```python
from build123d import *

# Parameters (mm, degrees)
F0_W     = 50.8
F0_H     = 19.05
F1_DEPTH = 19.05
F2_R     = 5.08
F3_R     = 5.08
F4_W     = 18.7399210408
F4_H     = 7.62
F5_DEPTH = 0.508
F6_R     = 0.1690866305
F6_R_2   = 0.254
F6_R_3   = 0.1908338751
F6_R_4   = 0.1508847562
F7_DEPTH = 0.254
F8_W     = 6.35
F8_H     = 5.08
F9_DEPTH = 50.8
F10_R    = 5.07999


# Not quite as in the source:
# - a fillet or chamfer is up to 0.001 mm smaller than in the source, because OpenCascade refuses the exact size


with BuildPart() as f1:
    # F0 (on Top) → F1 (new body)
    with BuildSketch(Plane.XY):
        Rectangle(F0_W, F0_H)
    extrude(amount=F1_DEPTH)

    # F2
    f2_edges = [f1.edges().sort_by_distance(p)[0] for p in [
        (-25.4, -9.525, 9.525),
        (25.4, -9.525, 9.525),
    ]]
    fillet(f2_edges, radius=F2_R)

    # F3
    f3_edges = [f1.edges().sort_by_distance(p)[0] for p in [
        (25.4, 2.54, 0),
    ]]
    fillet(f3_edges, radius=F3_R)

    # F4 (on face) → F5 (join)
    with BuildSketch(Plane.XZ.offset(9.525)):
        with Locations((0.5450607277, 15.24)):
            Rectangle(F4_W, F4_H)
    extrude(amount=F5_DEPTH)

    # F6 (on face) → F7 (join)
    with BuildSketch(Plane.XZ.offset(10.033)):
        with Locations((4.971065205, 13.6094420754)):
            Circle(F6_R)
        with Locations((-3.7048892478, 13.6058607324)):
            Circle(F6_R_2)
        with Locations((5.0740026747, 16.8156122121)):
            Circle(F6_R_3)
        with Locations((-3.7048892478, 16.8490853095)):
            Circle(F6_R_4)
    extrude(amount=F7_DEPTH)

    # F8 (on face) → F9 (cut)
    with BuildSketch(Plane.YZ.offset(25.4)):
        with Locations((6.35, 16.51)):
            Rectangle(F8_W, F8_H)
    extrude(amount=-F9_DEPTH, mode=Mode.SUBTRACT)

    # F10 (radius 5.08 in the source; OpenCascade refuses exactly that, so slightly less here)
    f10_edges = [f1.edges().sort_by_distance(p)[0] for p in [
        (0, 3.175, 13.97),
    ]]
    fillet(f10_edges, radius=F10_R)


solid = f1.part
```
The listing builds one solid part. Answer for the finished solid, in the listing's coordinates (mm). A direction names the side the tool comes from. Give positions to 0.01 mm unless a question says otherwise; leave off trailing zeros. Order: outer loops, then holes, each group sorted by start corner. A loop starts at its lowest first (then second) coordinate and runs counter-clockwise, first axis right, second up.
1) Find section C-C on y = 5.5. Write down the section's boundary in (x, z).
Reported:
outline: (-25.4, 5.08) arc R5.08 ccw to (-20.32, 0) - (20.32, 0) arc R5.08 ccw to (25.4, 5.08) - (25.4, 14.78) - (-25.4, 14.78) - close
2) Find section B-B on z = 12.75. Write down the section's boundary in (x, y) (3 decimals), then the cut area to 3 significant figures.
Reported:
outline: (-25.4, -4.445) arc R5.08 ccw to (-20.32, -9.525) - (-8.825, -9.525) - (-8.825, -10.033) - (9.915, -10.033) - (9.915, -9.525) - (20.32, -9.525) arc R5.08 ccw to (25.4, -4.445) - (25.4, 9.525) - (-25.4, 9.525) - close
area: 966 mm2
3) For faces 1 (the face through (0, 9, 13.97)), 2 (the face through (23.872, 2.638, 1.449)), determine the directions among +Z, -Z, +X, -X, +Y, -Y from which every point of the face is accessible in a straight line to the end or side of a thin tool.
Reported:
face 1: +Z, +X, -X, +Y
face 2: -Z, +X, +Y, -Y
4) Consider line 1 along Y through (x, z) = (-19.5, 5.75) (3 decimals); line 2 along Z through (x, y) = (17, -5.25); line 3 along Y through (x, z) = (-9.5, 1) (3 decimals). Determine where each line is inside the solid, lowest interval first.
Reported:
line 1: y = -9.525 to 9.525
line 2: z = 0.06 to 19.05
line 3: y = -7.472 to 9.525
5) Given P1, Ø1.4, axis at x = 4, y = 9, coming from the +Z side; P2, Ø3, axis at x = 17, y = 5.5, coming from the +Z side, each flat-ended and moving along its own axis, determine where each tip first touches the part or whether it passes through.
Reported:
P1: stops at z = 13.97
P2: stops at z = 16.27
